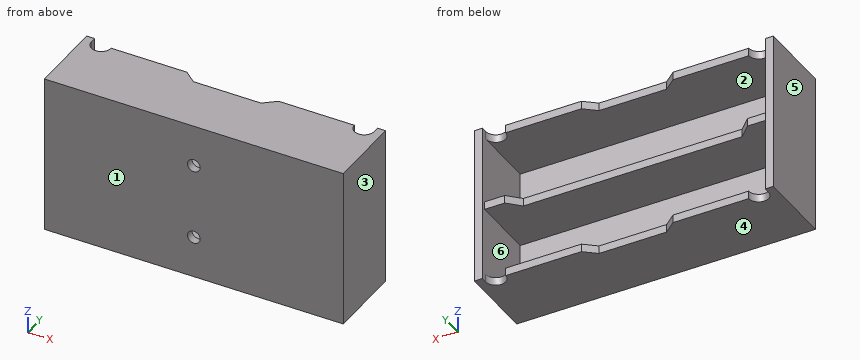
from build123d import *

# Parameters (mm, degrees)
SKETCH1_W           = 75
SKETCH1_H           = 40
BOSS_EXTRUDE1_DEPTH = 2
SKETCH2_W           = 75
SKETCH2_H           = 40
SKETCH2_W_2         = 71
SKETCH2_H_2         = 17
BOSS_EXTRUDE2_DEPTH = 17
CUT_EXTRUDE2_DEPTH  = 17
CUT_EXTRUDE3_REACH  = 82.169
CUT_EXTRUDE4_REACH  = 88.683
SKETCH5_R           = 1.6


with BuildPart() as part:
    # Sketch1 → Boss-Extrude1 (new body)
    with BuildSketch(Plane(origin=(0, 0, 0), x_dir=(1, 0, 0), z_dir=(0, 1, 0))):
        with Locations((37.5, 20)):
            Rectangle(SKETCH1_W, SKETCH1_H)
    extrude(amount=BOSS_EXTRUDE1_DEPTH)

    # Sketch2 → Boss-Extrude2 (add)
    with BuildSketch(Plane(origin=(0, 2, 0), x_dir=(1, 0, 0), z_dir=(0, 1, 0))):
        with Locations((37.5, 20)):
            Rectangle(SKETCH2_W, SKETCH2_H)
        with Locations((37.5, 29.5)):
            Rectangle(SKETCH2_W_2, SKETCH2_H_2, mode=Mode.SUBTRACT)
        with Locations((37.5, 10.5)):
            Rectangle(SKETCH2_W_2, SKETCH2_H_2, mode=Mode.SUBTRACT)
    extrude(amount=BOSS_EXTRUDE2_DEPTH)

    # Sketch3 → Cut-Extrude2 (cut)
    with BuildSketch(Plane.XY):
        with BuildLine():
            Line((2, 17.5), (2, 19))
            Line((2, 19), (73, 19))
            Line((73, 19), (73, 17.5))
            ThreePointArc((73, 17.5), (70.5, 15), (68, 17.5))
            Line((68, 17.5), (49, 17.5))
            Line((49, 17.5), (46, 15))
            Line((46, 15), (29, 15))
            Line((29, 15), (26, 17.5))
            Line((26, 17.5), (7, 17.5))
            ThreePointArc((7, 17.5), (4.5, 15), (2, 17.5))
        make_face()
    cut_extrude2 = extrude(amount=-CUT_EXTRUDE2_DEPTH, mode=Mode.SUBTRACT)

    # Mirror1: Cut-Extrude2 across plane
    add(cut_extrude2.mirror(Plane.XY.offset(-20)), mode=Mode.SUBTRACT)

    # Sketch4 → Cut-Extrude3 (cut, up to next)
    with BuildSketch(Plane.XY.offset(-19), mode=Mode.PRIVATE) as cut_extrude3_sk1:
        Polygon((2, 18), (7.035918341, 18), (10.035918341, 15), (64.964081659, 15), (67.964081659, 18), (73, 18), (73, 19), (2, 19), align=None)
    cut_extrude3_tool1 = extrude(cut_extrude3_sk1.sketch, amount=-CUT_EXTRUDE3_REACH, mode=Mode.PRIVATE) & part.part
    add(cut_extrude3_tool1.solids().sort_by_distance((37.5, 17.098486, -19))[0], mode=Mode.SUBTRACT)

    # Sketch5 → Cut-Extrude4 (cut, up to next)
    with BuildSketch(Plane(origin=(0, 2, 0), x_dir=(1, 0, 0), z_dir=(0, 1, 0)), mode=Mode.PRIVATE) as cut_extrude4_sk1:
        with Locations(Location((37.5, 29.5, 0), (0, 0, 270))):
            Circle(SKETCH5_R)
    cut_extrude4_tool1 = extrude(cut_extrude4_sk1.sketch, amount=-CUT_EXTRUDE4_REACH, mode=Mode.PRIVATE) & part.part
    # Sketch5 → Cut-Extrude4 (cut, up to next)
    with BuildSketch(Plane(origin=(0, 2, 0), x_dir=(1, 0, 0), z_dir=(0, 1, 0)), mode=Mode.PRIVATE) as cut_extrude4_sk2:
        with Locations(Location((37.5, 10.5, 0), (0, 0, 270))):
            Circle(SKETCH5_R)
    cut_extrude4_tool2 = extrude(cut_extrude4_sk2.sketch, amount=-CUT_EXTRUDE4_REACH, mode=Mode.PRIVATE) & part.part
    add(cut_extrude4_tool1.solids().sort_by_distance((37.5, 2, -29.5))[0], mode=Mode.SUBTRACT)
    add(cut_extrude4_tool2.solids().sort_by_distance((37.5, 2, -10.5))[0], mode=Mode.SUBTRACT)


solid = part.part
Could you check a few things on this model? Use its own coordinates, in mm. Face numbers are marked on the shaded views. A direction names the side the tool comes from. Coordinates: 2 decimals unless noted, no trailing zeros. Order: outer loops, then holes, each group sorted by start corner. A loop starts at its lowest first (then second) coordinate and runs counter-clockwise, first axis right, second up. Notation, with made-up numbers: (54.25, 22.5) - (110.25, 22.5) arc R21 ccw to (110.25, 46.5) - close; hole circle Ø3 at (10, 11.25). An arc over 180 degrees is marked (long way). Answer in a Markdown table with one row per item. Add a question column.
(1) If we section it at B-B, the plane x = 37.5: Please give me the cut outline in (y, z), then the cut area to 3 significant figures.
(2) If we section it at A-A, the plane z = -29.5: Please give me the cut outline in (x, y), then the cut area to 3 significant figures.
(3) On a 3-axis mill with a long thin cutter (end or side, diameter ignored), from which of +Z, -Z, +X, -X, +Y, -Y can I reach the whole of each face in a straight line? I mean the marked faces 1 and 2. Say none if no direction works.
(4) I need wall thicknesses on L1, parallel to Z at x = 37, y = 5.75; L2, parallel to X at y = 17.25, z = -11.5; L3, parallel to X at y = 0.65, z = -29.5. Which ranges of each line are inside material? Lowest first, please.
(5) If we section it at D-D, the plane z = -33.5: Please give me the cut outline in (x, y), then the cut area to 3 significant figures.
(6) Will these pins go through, and if not, where does the flat tip stop? pin 1 (1.6 mm diameter, centred on x = 60.5, z = -1, fed in from +Y); pin 2 (5 mm diameter, centred on x = 37.5, z = -10.5, fed in from +Y); pin 3 (0.6 mm diameter, centred on x = 70, z = -19.5, fed in from +Y); pin 4 (2.5 mm diameter, centred on x = 37.5, z = -29.5, fed in from -Y).
(7) If we mould it in two halves opening along X, with no side actions, what happens to the marked faces 3, 4, 5 and 6? For each: released by +X, released by -X, zero draft, split by the parting line, or undercut.
(8) If we section it at C-C, the plane y = 4.75: Please give me the cut outline in (x, z).
Results are:
| question | item | result |
|---|---|---|
| 1 | outline | (0, -40) - (15, -40) - (15, -38) - (2, -38) - (2, -31.1) - (0, -31.1) - close; (0, -27.9) - (2, -27.9) - (2, -21) - (15, -21) - (15, -19) - (2, -19) - (2, -12.1) - (0, -12.1) - close; (0, -8.9) - (2, -8.9) - (2, -2) - (15, -2) - (15, 0) - (0, 0) - close |
| 1 | area | 145 mm2 |
| 2 | outline | (0, 0) - (35.9, 0) - (35.9, 2) - (2, 2) - (2, 19) - (0, 19) - close; (39.1, 0) - (75, 0) - (75, 19) - (73, 19) - (73, 2) - (39.1, 2) - close |
| 2 | area | 212 mm2 |
| 3 | face 1 | +Z, -Z, +X, -X, -Y |
| 3 | face 2 | +Y |
| 4 | L1 | z = -40 to -38, -21 to -19, -2 to 0 |
| 4 | L2 | x = 0 to 2, 73 to 75 |
| 4 | L3 | x = 0 to 35.9, 39.1 to 75 |
| 5 | outline | (0, 0) - (75, 0) - (75, 19) - (73, 19) - (73, 2) - (2, 2) - (2, 19) - (0, 19) - close |
| 5 | area | 218 mm2 |
| 6 | pin 1 | stops at y = 17.5 |
| 6 | pin 2 | stops at y = 2 |
| 6 | pin 3 | stops at y = 18 |
| 6 | pin 4 | passes through |
| 7 | face 3 | released by +X |
| 7 | face 4 | zero draft |
| 7 | face 5 | released by -X |
| 7 | face 6 | undercut |
| 8 | outline | (0, -40) - (75, -40) - (75, 0) - (0, 0) - close; hole (2, -38) - (73, -38) - (73, -21) - (2, -21) - close; hole (2, -19) - (73, -19) - (73, -2) - (2, -2) - close |
